Read the model definition and answer for the solid it produces. Units are mm, in the model's axes. A direction names the side the tool comes from. Give positions to 0.01 mm unless a question says otherwise; leave off trailing zeros. Order: outer loops, then holes, each group sorted by start corner. A loop starts at its lowest first (then second) coordinate and runs counter-clockwise, first axis right, second up. Notation, with made-up numbers: (-18.5, 47.25) - (-11.5, 47.25) arc R37 cw to (-11.5, 86.25) - close; hole circle Ø5 at (84, 63). An arc over 180 degrees is marked (long way). Return JSON: item names as keys, results as strings.
```python
from build123d import *

# Parameters (mm, degrees)
BOSS_EXTRUDE1_DEPTH        = 27.22
CUT_EXTRUDE1_DEPTH         = 36.045677694
CUT_EXTRUDE1_DEPTH_BACK    = 2.5
SKETCH1_W                  = 37.05
SKETCH1_H                  = 20
F_2_8_2_8_DIAMETER_HOLE1_D = 2.8
FILLET3_R                  = 2.5
FILLET4_R                  = 1.25
F_3_8_3_8_DIAMETER_HOLE1_D = 3.8
FILLET5_R                  = 1.25


with BuildPart() as part:
    # Sketch2 → Boss-Extrude1 (new body)
    with BuildSketch(Plane(origin=(0, 11.515, 0), x_dir=(1, 0, 0), z_dir=(0, 1, 0))):
        Polygon((-27, 1.45), (-21.02, 1.45), (-21.02, 0), (21.02, 0), (21.02, 1.45), (29.5, 1.45), (29.5, -10.55), (27, -10.55), (27, -2.55), (-27, -2.55), align=None)
    extrude(amount=-BOSS_EXTRUDE1_DEPTH)

    # Sketch1 → Cut-Extrude1 (cut, two sides: drawn at the far end of the back side and taken through both)
    with BuildSketch(Plane.XY.offset(-CUT_EXTRUDE1_DEPTH_BACK)):
        Rectangle(SKETCH1_W, SKETCH1_H)
    extrude(amount=CUT_EXTRUDE1_DEPTH + CUT_EXTRUDE1_DEPTH_BACK, mode=Mode.SUBTRACT)

    # Ø2.8 (2.8) Diameter Hole1 (through all)
    with Locations(Plane.XY.offset(2.55)):
        with Locations((24, -12.705), (-24, -12.705), (-24, 8.515), (24, 8.515)):
            Hole(F_2_8_2_8_DIAMETER_HOLE1_D / 2)

    # Fillet3
    fillet3_edges = [part.edges().sort_by_distance(p)[0] for p in [
        (-27, 11.515, 0.55),
        (29.5, -2.095, -1.45),
        (-27, -15.705, 0.55),
    ]]
    fillet(fillet3_edges, radius=FILLET3_R)

    # Fillet4
    fillet4_edges = [part.edges().sort_by_distance(p)[0] for p in [
        (27, -2.095, 2.55),
    ]]
    fillet(fillet4_edges, radius=FILLET4_R)

    # Ø3.8 (3.8) Diameter Hole1 (through all)
    with Locations(Plane(origin=(29.5, 0, 0), x_dir=(0, 0, -1), z_dir=(1, 0, 0))):
        with Locations((-6.05, -9.595), (-6.05, 5.405)):
            Hole(F_3_8_3_8_DIAMETER_HOLE1_D / 2)

    # Fillet5
    fillet5_edges = [part.edges().sort_by_distance(p)[0] for p in [
        (28.25, 11.515, 10.55),
        (28.25, -15.705, 10.55),
    ]]
    fillet(fillet5_edges, radius=FILLET5_R)


solid = part.part
```
Q1. Determine the mould class of faces 4 (the cylindrical face through (28.23, -7.71, 5.8)), 5 (the flat face through (0, 10, 1)), 6 (the cylindrical face through (28.748, -2.286, -0.737)) for opening direction Z: released by +Z, released by -Z, zero draft, split by the parting line, or undercut.
Values:
{"face 4": "undercut", "face 5": "zero draft", "face 6": "released by -Z"}
Q2. A cutting plane is placed at B-B (z = 6.05). Write down the section's boundary in (x, y) (3 decimals).
Values:
{"outline": "(27, -15.705) - (29.5, -15.705) - (29.5, -11.495) - (27, -11.495) - close; (27, -7.695) - (29.5, -7.695) - (29.5, 3.505) - (27, 3.505) - close; (27, 7.305) - (29.5, 7.305) - (29.5, 11.515) - (27, 11.515) - close"}
Q3. A cutting plane is placed at C-C (y = -0.25). Write down the section's boundary in (x, z) (3 decimals), and give its area (3 significant figures).
Values:
{"outline": "(-27, -1.45) - (-21.02, -1.45) - (-21.02, 0) - (-18.525, 0) - (-18.525, 2.55) - (-27, 2.55) - close; (18.525, 0) - (21.02, 0) - (21.02, -1.45) - (27, -1.45) arc R2.5 ccw to (29.5, 1.05) - (29.5, 10.55) - (27, 10.55) - (27, 3.8) arc R1.25 cw to (25.75, 2.55) - (18.525, 2.55) - close", "area": "89.6 mm²"}
Q4. A cutting plane is placed at A-A (x = 24). Write down the section's boundary in (y, z) (3 decimals), and give its area (3 significant figures).
Values:
{"outline": "(-15.705, -1.45) - (-14.105, -1.45) - (-14.105, 2.55) - (-15.705, 2.55) - close; (-11.305, -1.45) - (7.115, -1.45) - (7.115, 2.55) - (-11.305, 2.55) - close; (9.915, -1.45) - (11.515, -1.45) - (11.515, 2.55) - (9.915, 2.55) - close", "area": "86.5 mm²"}
Q5. For faces 1 (the flat face through (0, -10, 1)), 2 (the flat face through (-5, -11, 0)), 3 (the cylindrical face through (-26.29, -14.95, 0.52)), determine the directions among +Z, -Z, +X, -X, +Y, -Y from which every point of the face is accessible in a straight line to the end or side of a thin tool.
Values:
{"face 1": "+Z, -Z", "face 2": "-Z, +Y, -Y", "face 3": "+Z, -Z, -X, -Y"}
Q6. Given pin 1 (13.5 mm diameter, centred on x = 0, y = -5.5, fed in from -Z); pin 2 (6 mm diameter, centred on y = 5.405, z = 6.05, fed in from -X); pin 3 (3 mm diameter, centred on x = 24, y = -12.705, fed in from +Z), each flat-ended and moving along its own axis, determine where each tip first touches the part or whether it passes through.
Values:
{"pin 1": "stops at z = 0", "pin 2": "stops at x = 26.75", "pin 3": "stops at z = 2.55"}
Q7. Consider L1, parallel to Y at x = 24, z = 0 (3 decimals); L2, parallel to Y at x = 28.85, z = 6.05 (3 decimals); L3, parallel to Y at x = 7.5, z = 2 (3 decimals). Determine where each line is inside the solid, lowest interval first.
Values:
{"L1": "y = -15.705 to -14.105, -11.305 to 7.115, 9.915 to 11.515", "L2": "y = -15.705 to -11.495, -7.695 to 3.505, 7.305 to 11.515", "L3": "y = -15.705 to -10, 10 to 11.515"}
Q8. A cutting plane is placed at D-D (x = -15). Write down the section's boundary in (y, z) (3 decimals).
Values:
{"outline": "(-15.705, 0) - (-10, 0) - (-10, 2.55) - (-15.705, 2.55) - close; (10, 0) - (11.515, 0) - (11.515, 2.55) - (10, 2.55) - close"}
